Geometry: final body of the model. Coordinates: model frame, mm. Round coordinates to 2 decimals unless told otherwise and drop trailing zeros. Loops run counter-clockwise (first coordinate to the right, second up) from the corner with the lowest first, then second, coordinate; pieces in that order, holes last. Notation, with made-up numbers: (-22.75, 61.25) - (16.25, 61.25) arc R29 cw to (16.25, 82.25) - close; hole circle Ø5 at (52, 88). An arc over 180 degrees is marked (long way). Answer as a JSON object with one key per item and string values. Group by question number.
Item 1: Line query: line 1 (X direction, y = 2.1, z = -26.5); line 2 (X direction, y = 0.8, z = -40); line 3 (Z direction, x = -2, y = 0.95). Output: solid intervals per line, ascending.
Item 2: First-contact query: pin 1 (1.8 mm diameter, centred on x = 92.76, z = 48.98, fed in from -Y); pin 2 (1.5 mm diameter, centred on x = -65.5, y = 1.5, fed in from +Z); pin 3 (1.5 mm diameter, centred on x = -34, y = 2, fed in from +Z). Flat tips, straight axial feed; report the tip coordinate or a pass-through.
Item 3: Draft query along X for faces 1 (the face through (-65.4, 1.52, -49.46)), 2 (the face through (-67.69, 1.52, 51.4)), 3 (the face through (2, 0, 2)). Return one class per face: released by +X, released by -X, zero draft, split by the parting line, or undercut.
Item 4: Section B-B (z = -14). Return the cut outline in (x, y).
Item 5: Section A-A (y = 1.1). Count the separate pieces of the cut face and the enclosed holes in it, plus the area to 3 significant figures.
Item 6: Section C-C (x = -57.5). Return the cut outline in (y, z).
```python
from build123d import *

# Parameters (mm, degrees)
SKETCH1_R               = 1.5
BOSS_EXTRUDE1_DEPTH     = 3
CUT_EXTRUDE1_DEPTH      = 117.441839515
CUT_EXTRUDE1_DEPTH_BACK = 117.441839515
BOSS_EXTRUDE4_DEPTH     = 3
SKETCH5_W               = 197.044523164
SKETCH5_H               = 3
BOSS_EXTRUDE5_DEPTH     = 3
CUT_EXTRUDE3_DEPTH      = 117.441839515
CUT_EXTRUDE3_DEPTH_BACK = 117.441839515
SKETCH6_R               = 2


with BuildPart() as part:
    # Sketch1 → Boss-Extrude1 (new body)
    with BuildSketch(Plane(origin=(0, 0, 0), x_dir=(1, 0, 0), z_dir=(0, 1, 0))):
        Polygon((-84.458557919, 26.833968268), (-84.458557919, 48.772574994), (-94.458442431, 48.8206348), (-94.578591945, 23.820923519), (-94.881368721, -39.178348907), (-94.952977831, -54.07817683), (98.36173931, -55.007254334), (102.586080733, -55.007254334), (102.586080733, 22.87334299), (102.586080733, 48.772574994), (-62.665629197, 48.772574994), (-62.665629197, 26.833968268), align=None)
        with Locations(Location((-89.851389086, -34.95245099, 0), (0, 0, 270))):
            Circle(SKETCH1_R, mode=Mode.SUBTRACT)
        with Locations(Location((-1.069960941, -29.129088653, 0), (0, 0, 270))):
            Circle(SKETCH1_R, mode=Mode.SUBTRACT)
        with Locations(Location((-89.791314329, -22.452595349, 0), (0, 0, 270))):
            Circle(SKETCH1_R, mode=Mode.SUBTRACT)
        with Locations(Location((-48.61901855, -28.900566167, 0), (0, 0, 270))):
            Circle(SKETCH1_R, mode=Mode.SUBTRACT)
        with Locations(Location((78.109513121, -48.909852111, 0), (0, 0, 270))):
            Circle(SKETCH1_R, mode=Mode.SUBTRACT)
        with Locations(Location((92.757382127, -48.980250297, 0), (0, 0, 270))):
            Circle(SKETCH1_R, mode=Mode.SUBTRACT)
        with Locations(Location((-89.548612311, 30.046821437, 0), (0, 0, 270))):
            Circle(SKETCH1_R, mode=Mode.SUBTRACT)
        with Locations(Location((-89.488537553, 42.546677077, 0), (0, 0, 270))):
            Circle(SKETCH1_R, mode=Mode.SUBTRACT)
        with Locations(Location((-48.297017852, 38.098660064, 0), (0, 0, 270))):
            Circle(SKETCH1_R, mode=Mode.SUBTRACT)
        with Locations(Location((-0.747960243, 37.870137578, 0), (0, 0, 270))):
            Circle(SKETCH1_R, mode=Mode.SUBTRACT)
        with Locations(Location((77.015212266, 28.9963068, 0), (0, 0, 270))):
            Circle(SKETCH1_R, mode=Mode.SUBTRACT)
        with Locations(Location((91.576164691, 31.240232702, 0), (0, 0, 270))):
            Circle(SKETCH1_R, mode=Mode.SUBTRACT)
    extrude(amount=BOSS_EXTRUDE1_DEPTH)

    # Sketch3 → Cut-Extrude1 (cut, two sides: drawn at the far end of the back side and taken through both)
    with BuildSketch(Plane(origin=(0, 3, 0), x_dir=(1, 0, 0), z_dir=(0, 1, 0)).offset(-CUT_EXTRUDE1_DEPTH_BACK)):
        Polygon((-62.665629197, 26.833968268), (-77.458442431, 26.833968268), (-77.458442431, 10.8206348), (-54.548666479, 10.8206348), (-54.548666479, 48.772574994), (-62.665629197, 48.772574994), align=None)
    extrude(amount=CUT_EXTRUDE1_DEPTH + CUT_EXTRUDE1_DEPTH_BACK, mode=Mode.SUBTRACT)

    # Sketch4 → Boss-Extrude4 (add)
    with BuildSketch(Plane.XZ):
        Polygon((-77.458442431, -26.833968268), (-84.458557919, -26.833968268), (-84.458557919, -48.772574994), (-54.548666479, -48.772574994), (-54.548666479, -43.333568131), (-77.458442431, -43.333568131), align=None)
    extrude(amount=-BOSS_EXTRUDE4_DEPTH)

    # Sketch5 → Boss-Extrude5 (add)
    with BuildSketch(Plane.XZ):
        with Locations((4.063819151, -50.272574994)):
            Rectangle(SKETCH5_W, SKETCH5_H)
    extrude(amount=-BOSS_EXTRUDE5_DEPTH)

    # Sketch6 → Cut-Extrude3 (cut, two sides: drawn at the far end of the back side and taken through both)
    with BuildSketch(Plane.XZ.offset(-CUT_EXTRUDE3_DEPTH_BACK)):
        with Locations(Location((-66.003554455, -47.553071563, 0), (0, 0, 270))):
            Circle(SKETCH6_R)
        with Locations(Location((62.548576351, -47.553071563, 0), (0, 0, 90))):
            Circle(SKETCH6_R)
        with Locations(Location((62.548576351, 50.323212151, 0), (0, 0, 270))):
            Circle(SKETCH6_R)
        with Locations(Location((-66.003554455, 50.323212151, 0), (0, 0, 90))):
            Circle(SKETCH6_R)
    extrude(amount=CUT_EXTRUDE3_DEPTH + CUT_EXTRUDE3_DEPTH_BACK, mode=Mode.SUBTRACT)


solid = part.part
```
Values:
{
 "1": {"line 1": "x = -94.57 to -77.46, -54.55 to 102.59", "line 2": "x = -94.5 to -77.46, -54.55 to 102.59", "line 3": "z = -51.77 to -38.7, -37.04 to 27.95, 30.31 to 54.52"},
 "2": {"pin 1": "passes through", "pin 2": "stops at z = 54.22", "pin 3": "stops at z = 54.37"},
 "3": {"face 1": "undercut", "face 2": "undercut", "face 3": "zero draft"},
 "4": {"outline": "(-94.63, 0) - (-77.46, 0) - (-77.46, 3) - (-94.63, 3) - close; (-54.55, 0) - (102.59, 0) - (102.59, 3) - (-54.55, 3) - close"},
 "5": {"separate pieces": "1", "enclosed holes": "17", "area": "20,100 mm^2"},
 "6": {"outline": "(0, -51.77) - (3, -51.77) - (3, -43.33) - (0, -43.33) - close; (0, -10.82) - (3, -10.82) - (3, 54.26) - (0, 54.26) - close"}
}
